from build123d import *

# Parameters (mm, degrees)
ESQUISSE2_R             = 2.1
BOSS_EXTRU_1_DEPTH      = 18
ENL_V_START             = -6.8
ESQUISSE3_R             = 13.4
ESQUISSE3_R_2           = 13.35
ENL_V_MAT_EXTRU_1_DEPTH = 0.8


with BuildPart() as part:
    # Esquisse1 → Révolution1 (revolve)
    with BuildSketch(Plane.XY, mode=Mode.PRIVATE) as r_volution1_sk:
        Polygon((-33.6, 0), (-33.6, 2.15), (-26.8, 2.15), (-26.8, 13.4), (0, 13.4), (0, 12.1), (30.8, 12.1), (30.8, 3.1), (33.1, 3.1), (33.1, 0), align=None)
    revolve(r_volution1_sk.sketch.rotate(Axis((0, 0, 0), (1, 0, 0)), 90), axis=Axis((0, 0, 0), (1, 0, 0)))

    # Esquisse2 → Boss.-Extru.1 (add)
    with BuildSketch(Plane(origin=(0, 0, 0), x_dir=(1, 0, 0), z_dir=(0, 1, 0))):
        with Locations(Location((-6, 0, 0), (0, 0, 90))):
            Circle(ESQUISSE2_R)
    extrude(amount=BOSS_EXTRU_1_DEPTH)

    # Esquisse3 → Enlèv. mat.-Extru.1 (cut)
    with BuildSketch(Plane.ZY.offset(26.8).offset(ENL_V_START)):
        Circle(ESQUISSE3_R)
        Circle(ESQUISSE3_R_2, mode=Mode.SUBTRACT)
    extrude(amount=ENL_V_MAT_EXTRU_1_DEPTH, mode=Mode.SUBTRACT)


solid = part.part
Source: CAD feature listing. Evaluate the final solid. Frame: model axes, mm. A direction names the side the tool comes from. Round coordinates to 2 decimals unless told otherwise and drop trailing zeros. Loops run counter-clockwise (first coordinate to the right, second up) from the corner with the lowest first, then second, coordinate; pieces in that order, holes last. Notation, with made-up numbers: (82, 52.25) - (137, 52.25) arc R27 cw to (137, 85.25) - close; hole circle Ø2 at (-34, -20.75). An arc over 180 degrees is marked (long way). Write item = value, one per line. Start each with the question number.
(1) Section query B-B, the plane y = 0. Output: boundary loops of the cut face in (x, z).
(2) Pin query (flat end, axial travel): pin 1 (1.5 mm diameter, centred on x = 17, z = -8.5, fed in from +Y); pin 2 (5 mm diameter, centred on y = 10.5, z = -10.5, fed in from +X); pin 3 (10 mm diameter, centred on x = 24, y = -1, fed in from +Z); pin 4 (5 mm diameter, centred on y = 12, z = 10.5, fed in from +X). Return the tip coordinate at first contact, or that it passes through.
(3) Section query C-C, the plane x = -24.5. Output: boundary loops of the cut face in (y, z), plus the area to 3 significant figures.
(4) Section query D-D, the plane y = 8.5. Output: boundary loops of the cut face in (x, z).
(5) Set-up query: faces 1 (the face through (30.8, 3, 3)), 2 (the face through (-20.394, 4.01, 12.734)), 3 (the face through (-30.15, -0.09, -2.15)), 4 (the face through (-8.082, 15.582, 0.273)). Return all of +Z, -Z, +X, -X, +Y, -Y with unobstructed straight access to the full face (end or side cutting, diameter ignored); none if empty.
(6) Section query A-A, the plane z = 0. Output: boundary loops of the cut face in (x, y).
(7) Ray query, line 1 along X through (y, z) = (-5.5, 11.25); line 2 along X through (y, z) = (6, 2.5); line 3 along Y through (x, z) = (-16, 6.5). Return the intervals inside material, ascending. Write a range as from..to.
Conclusion:
q1.outline = (-33.6, -2.15) - (-26.8, -2.15) - (-26.8, -13.4) - (-20.8, -13.4) - (-20.8, -13.35) - (-20, -13.35) - (-20, -13.4) - (0, -13.4) - (0, -12.1) - (30.8, -12.1) - (30.8, -3.1) - (33.1, -3.1) - (33.1, 3.1) - (30.8, 3.1) - (30.8, 12.1) - (0, 12.1) - (0, 13.4) - (-20, 13.4) - (-20, 13.35) - (-20.8, 13.35) - (-20.8, 13.4) - (-26.8, 13.4) - (-26.8, 2.15) - (-33.6, 2.15) - close
q2.pin_1 = 9.29
q2.pin_2 = 0
q2.pin_3 = 12.1
q2.pin_4 = through
q3.outline = circle Ø26.8 at (0, 0)
q3.area = 564 mm2
q4.outline = (-26.8, -10.36) - (-20.8, -10.36) - (-20.8, -10.29) - (-20, -10.29) - (-20, -10.36) - (0, -10.36) - (0, -8.61) - (30.8, -8.61) - (30.8, 8.61) - (0, 8.61) - (0, 10.36) - (-20, 10.36) - (-20, 10.29) - (-20.8, 10.29) - (-20.8, 10.36) - (-26.8, 10.36) - close
q5.face_1 = +X
q5.face_2 = none
q5.face_3 = -X
q5.face_4 = +Y
q6.outline = (-33.6, -2.15) - (-26.8, -2.15) - (-26.8, -13.4) - (-20.8, -13.4) - (-20.8, -13.35) - (-20, -13.35) - (-20, -13.4) - (0, -13.4) - (0, -12.1) - (30.8, -12.1) - (30.8, -3.1) - (33.1, -3.1) - (33.1, 3.1) - (30.8, 3.1) - (30.8, 12.1) - (0, 12.1) - (0, 13.4) - (-3.9, 13.4) - (-3.9, 18) - (-8.1, 18) - (-8.1, 13.4) - (-20, 13.4) - (-20, 13.35) - (-20.8, 13.35) - (-20.8, 13.4) - (-26.8, 13.4) - (-26.8, 2.15) - (-33.6, 2.15) - close
q7.line_1 = -26.8..0
q7.line_2 = -26.8..30.8
q7.line_3 = -11.72..11.72
